```python
from build123d import *

# Parameters (mm, degrees)
SKETCH017_R     = 1.8
PAD008_DEPTH    = 18
SKETCH018_W     = 32
SKETCH018_H     = 6
POCKET_DEPTH    = 10.5
POCKET001_DEPTH = 14.051
POCKET002_DEPTH = 2.25
SKETCH_W        = 39.26252
SKETCH_H        = 23.934808
POCKET003_DEPTH = 0.5


with BuildPart() as part:
    # Sketch017 → Pad008 (new body)
    with BuildSketch(Plane.YZ):
        with BuildLine():
            Line((-16, 2.25), (-16, 0))
            Line((-16, 0), (-16, -5.8))
            Line((-16, -5.8), (-16, -11.8))
            Line((-16, -11.8), (16, -11.8))
            Line((16, -11.8), (16, -5.8))
            Line((16, -5.8), (16, 0))
            Line((16, 0), (16, 2.25))
            Line((14.0798989873, 2.25), (16, 2.25))
            ThreePointArc((14.0798989873, 2.25), (12.1, 2.95), (10.1201010127, 2.25))
            Line((10.1201010127, 2.25), (-10.1201010127, 2.25))
            ThreePointArc((-10.1201010127, 2.25), (-12.1, 2.95), (-14.0798989873, 2.25))
            Line((-14.0798989873, 2.25), (-16, 2.25))
        make_face()
        with Locations((-7, -8.9)):
            Circle(SKETCH017_R, mode=Mode.SUBTRACT)
        with Locations((7, -8.9)):
            Circle(SKETCH017_R, mode=Mode.SUBTRACT)
        with Locations((-12.1, -0.2)):
            Circle(SKETCH017_R, mode=Mode.SUBTRACT)
        with Locations((12.1, -0.2)):
            Circle(SKETCH017_R, mode=Mode.SUBTRACT)
    extrude(amount=-PAD008_DEPTH)

    # Sketch018 (on Face17 of Pad008) → Pocket (cut)
    with BuildSketch(Plane.YZ):
        with Locations((0, -8.8)):
            Rectangle(SKETCH018_W, SKETCH018_H)
    extrude(amount=-POCKET_DEPTH, mode=Mode.SUBTRACT)

    # Sketch019 (on Face3 of Pocket) → Pocket001 (cut, through all)
    with BuildSketch(Plane(origin=(0, 0, 2.25), x_dir=(0, -1, 0), z_dir=(0, 0, 1))):
        with BuildLine():
            ThreePointArc((-6.2, 0), (0, -6.2), (6.2, 0))
            Line((-6.2, 0), (6.2, 0))
        make_face()
    extrude(amount=-POCKET001_DEPTH, mode=Mode.SUBTRACT)

    # Sketch020 (on Face3 of Pocket001) → Pocket002 (cut)
    with BuildSketch(Plane(origin=(0, 0, 2.25), x_dir=(0, -1, 0), z_dir=(0, 0, 1))):
        with BuildLine():
            ThreePointArc((-8.2, 0), (0, -8.2), (8.2, 0))
            Line((-8.2, 0), (8.2, 0))
        make_face()
    extrude(amount=-POCKET002_DEPTH, mode=Mode.SUBTRACT)

    # Sketch (on Face8 of Pocket002) → Pocket003 (cut)
    with BuildSketch(Plane.YZ):
        with Locations((0.008158, -3.713083)):
            Rectangle(SKETCH_W, SKETCH_H)
    extrude(amount=-POCKET003_DEPTH, mode=Mode.SUBTRACT)


solid = part.part
```
Design review of the part built by this model. Coordinates are the model's own, in mm. A direction names the side the tool comes from. Coordinates: 2 decimals unless noted, no trailing zeros. Write each loop counter-clockwise with the first axis right and the second up, starting at its lowest first coordinate (ties: lowest second). Pieces come first, ordered by that corner, then holes.
1) Machinability: for faces 1 (the flat face through (-7, 0, 0)), 2 (the flat face through (-11, 0, 2.25)), 3 (the flat face through (-9, -15, 2.25)), which of the approach directions +Z, -Z, +X, -X, +Y, -Y give a long, thin tool a straight path to every point of the face, cutting with its end or side? Answer none if there is none.
2) Add section C-C (x = -9.25). Write out the cut boundary in (y, z).
3) Add section A-A (x = -3.25). Write out the cut boundary in (y, z), plus the area to 3 significant figures.
4) Mouldability with a two-part tool opening along Z and no side actions: class faces 4 (the cylindrical face through (-9.128, 13.763, -0.889)), 5 (the flat face through (-18, 0, -4)), 6 (the flat face through (-14, 0, -11.8)) as +Z half, -Z half, draft (parallel to the pull), parting line (faces both ways), or undercut.
5) Add section D-D (z = -1.25). Write out the cut boundary in (x, y).
6) To check wall thickness, follow L1, parallel to Z at x = -13.5, y = -7; L2, parallel to Z at x = -11.75, y = 12.1; L3, parallel to X at y = -2, z = -9. State the ranges of each line that lie inside material, in increasing order.
7) Add section B-B (y = 12.1). Write out the cut boundary in (x, z), plus the area to 3 significant figures.
8) Insertion check: pin 1 (8 mm diameter, centred on x = -3, y = 0.5, fed in from -Z); pin 2 (3 mm diameter, centred on y = -7.5, z = -8.5, fed in from +X); pin 3 (2 mm diameter, centred on x = -9.5, y = -15.5, fed in from +Z). Each pin has a flat end and moves straight along its axis. Give the tip position at first contact, or say it passes through.
Check result:
1. face 1: +Z, +X
1. face 2: +Z, +X, -X
1. face 3: +Z, +X, -X, -Y
2. outline: (-16, -5.8) - (16, -5.8) - (16, 2.25) - (14.08, 2.25) arc R3.15 ccw to (10.12, 2.25) - (-10.12, 2.25) arc R3.15 ccw to (-14.08, 2.25) - (-16, 2.25) - close; hole circle Ø3.6 at (-12.1, -0.2); hole circle Ø3.6 at (12.1, -0.2)
3. outline: (-16, -5.8) - (-5.28, -5.8) - (-5.28, 0) - (-7.53, 0) - (-7.53, 2.25) - (-10.12, 2.25) arc R3.15 ccw to (-14.08, 2.25) - (-16, 2.25) - close; (5.28, -5.8) - (16, -5.8) - (16, 2.25) - (14.08, 2.25) arc R3.15 ccw to (10.12, 2.25) - (7.53, 2.25) - (7.53, 0) - (5.28, 0) - close; hole circle Ø3.6 at (-12.1, -0.2); hole circle Ø3.6 at (12.1, -0.2)
3. area: 146 mm2
4. face 4: undercut
4. face 5: draft
4. face 6: -Z half
5. outline: (-18, -16) - (-0.5, -16) - (-0.5, -13.56) - (-18, -13.56) - close; (-18, -10.64) - (-0.5, -10.64) - (-0.5, -6.18) arc R6.2 cw to (-0.5, 6.18) - (-0.5, 10.64) - (-18, 10.64) - close; (-18, 13.56) - (-0.5, 13.56) - (-0.5, 16) - (-18, 16) - close
6. L1: z = -11.8 to -10.7, -7.1 to 2.25
6. L2: z = -11.8 to -2, 1.6 to 2.95
6. L3: x = -18 to -10.5
7. outline: (-18, -11.8) - (-10.5, -11.8) - (-10.5, -5.8) - (-0.5, -5.8) - (-0.5, -2) - (-18, -2) - close; (-18, 1.6) - (-0.5, 1.6) - (-0.5, 2.95) - (-18, 2.95) - close
7. area: 135 mm2
8. pin 1: stops at z = -5.8
8. pin 2: stops at x = -10.5
8. pin 3: stops at z = 2.25
